Could you check a few things on this model? Use its own coordinates, in mm. Face numbers are marked on the shaded views. A direction names the side the tool comes from. Coordinates: 2 decimals unless noted, no trailing zeros. Loops run counter-clockwise (first coordinate to the right, second up) from the corner with the lowest first, then second, coordinate; pieces in that order, holes last. Notation, with made-up numbers: (46.25, 21) -> (66.25, 21) arc R15 ccw to (66.25, 47) -> close; hole circle Ø5 at (20, 33). An arc over 180 degrees is marked (long way). One line per question, with ' | ' between items. Start each with the question number.
(1) I'm going to push flat-ended pins straight in: pin 1 Ø8 at (x, z) = (-11, 19) entering from -Y; pin 2 Ø7 at (y, z) = (-12, -36) entering from +X; pin 3 Ø10 at (y, z) = (-12, 4.5) entering from +X; pin 4 Ø2 at (x, y) = (-43.5, -7.5) entering from -Z. Where does each tip first touch, or does it pass through?
(2) Suppose I cut it at C-C (y = -16.5). Please give me the cut outline in (x, z).
(3) If I drill on line 1 along Y through (x, z) = (-49.5, 34); line 2 along X through (y, z) = (-4.5, 5); line 3 along X through (y, z) = (-25.5, 32), over which ranges is the centre line in solid material (lowest first)?
(4) Suppose I cut it at D-D (z = -35.5). Please give me the cut outline in (x, y).
(5) If we mould it in two halves opening along Z, with no side actions, what happens to the marked faces 1, 2 and 3? For each: pulls with the +Z half, pulls with the -Z half, needs draft (parallel to the pull), parting line crosses it, or undercut.
(6) Which directions (+Z, -Z, +X, -X, +Y, -Y) give clear straight access to the entire face, cutting with the end or side of a thin tool? Please do the marked faces 4, 5, 6 and 7.
(7) Suppose I cut it at B-B (z = 31). Please give me the cut outline in (x, y).
(8) Suppose I cut it at A-A (y = -25). Please give me the cut outline in (x, z) (3 decimals).
```python
from build123d import *

# Parameters (mm, degrees)
F0_W         = 130.5194124579
F0_H         = 87.0954208076
F1_DEPTH     = 5.08
F2_W         = 18.4217169881
F2_H         = 20.1326627284
F3_DEPTH     = 25.4
F4_W         = 18.0227532983
F4_H         = 20.2161408961
F5_DEPTH     = 25.4
F6_W         = 17.5940208137
F6_H         = 28.6207161844
F7_DEPTH     = 25.4
F8_T         = 2.54
F8_T3_DEPTH  = 22.6740208137
F8_T5_DEPTH  = 23.1027532983
F8_T7_DEPTH  = 25.2961408961
F8_T9_DEPTH  = 23.5017169881
F8_T11_DEPTH = 25.2126627284
F9_W         = 15.0540208137
F9_H         = 4.0768496692
F10_DEPTH    = 5.08
F11_W        = 26.8854014575
F11_H        = 26.7390697263
F12_DEPTH    = 2.54
F13_T1_DEPTH = 48.8824467137
F13_T3_DEPTH = 48.7361149824


# Not quite as in the source:
# - a fillet or chamfer that OpenCascade refuses, or shapes differently, is made with other operations: its cross-section is extruded or revolved along the edge and cut away or added
# - a shell that OpenCascade refuses in one call is made with other operations: the cavity is built on its own and cut out


with BuildPart() as f1:
    # F0 (on Front) → F1 (new body)
    with BuildSketch(Plane.XZ):
        with Locations((2.1416731179, -2.8366688639)):
            Rectangle(F0_W, F0_H)
    extrude(amount=F1_DEPTH)

    # F2 (on face) → F3 (join)
    with BuildSketch(Plane.XZ.offset(5.08)):
        with Locations((-53.9071746171, 30.6447101757)):
            Rectangle(F2_W, F2_H)
    extrude(amount=F3_DEPTH)

    # F4 (on face) → F5 (join)
    with BuildSketch(Plane.XZ.offset(5.08)):
        with Locations((-54.106656462, 0.4099132493)):
            Rectangle(F4_W, F4_H)
    extrude(amount=F5_DEPTH)

    # F6 (on face) → F7 (join)
    with BuildSketch(Plane.XZ.offset(5.08)):
        with Locations((-54.3210227042, -32.0740211755)):
            Rectangle(F6_W, F6_H)
    extrude(amount=F7_DEPTH)

    # F8: shell of thickness 2.54, made by hand


with BuildPart() as f8_core1:
    # F8_t2: copy of F1
    add(f1.part)

    # the walls: a layer under each face that stays
    f8_faces = [f8_core1.faces().sort_by_distance(p)[0] for p in [
        (-63.1180331111, -15.24, -2.8366688639),
        (2.1416731179, 0, -2.8366688639),
        (67.4013793468, -2.54, -2.8366688639),
        (-53.7952179355, -28.3028571429, -46.3843792677),
        (-54.3210227042, -30.48, -32.0740211755),
        (-54.3210227042, -17.78, -17.7636630833),
        (-54.106656462, -17.78, -9.6981571987),
        (-45.0952798128, -17.78, 0.4099132493),
        (-54.106656462, -30.48, 0.4099132493),
        (-54.106656462, -17.78, 10.5179836974),
        (2.1416731179, -5.08, -2.8366688639),
        (-44.696316123, -17.78, 30.6447101757),
        (-53.9071746171, -17.78, 20.5783788115),
        (-53.9071746171, -30.48, 30.6447101757),
        (58.0785641713, -2.1771428571, 40.7110415399),
    ]]
    thicken(f8_faces, amount=-F8_T, mode=Mode.SUBTRACT)

    # F8_s4 → F8_t3 (cut)
    with BuildSketch(Plane.YZ.offset(-65.6580331111)):
        Polygon((-5.1054, -17.7382630833), (-5.08, -20.3036630833), (-2.54, -20.3036630833), (-2.54, -17.7636630833), align=None)
    extrude(amount=F8_T3_DEPTH, mode=Mode.SUBTRACT)

    # F8_s6 → F8_t5 (cut)
    with BuildSketch(Plane.YZ.offset(-65.6580331111)):
        Polygon((-5.1054, -9.7235571987), (-5.08, -7.1581571987), (-2.54, -7.1581571987), (-2.54, -9.6981571987), align=None)
        Polygon((-5.1054, 10.5433836974), (-5.08, 7.9779836974), (-2.54, 7.9779836974), (-2.54, 10.5179836974), align=None)
    extrude(amount=F8_T5_DEPTH, mode=Mode.SUBTRACT)

    # F8_s8 → F8_t7 (cut)
    with BuildSketch(Plane.XY.offset(-12.2381571987)):
        Polygon((-45.0698798128, -5.1054), (-47.6352798128, -5.08), (-47.6352798128, -2.54), (-45.0952798128, -2.54), align=None)
    extrude(amount=F8_T7_DEPTH, mode=Mode.SUBTRACT)

    # F8_s10 → F8_t9 (cut)
    with BuildSketch(Plane.YZ.offset(-65.6580331111)):
        Polygon((-5.1054, 20.5529788115), (-2.54, 20.5783788115), (-2.54, 23.1183788115), (-5.08, 23.1183788115), align=None)
    extrude(amount=F8_T9_DEPTH, mode=Mode.SUBTRACT)

    # F8_s12 → F8_t11 (cut)
    with BuildSketch(Plane.XY.offset(18.0383788115)):
        Polygon((-44.670916123, -5.1054), (-44.696316123, -2.54), (-47.236316123, -2.54), (-47.236316123, -5.08), align=None)
    extrude(amount=F8_T11_DEPTH, mode=Mode.SUBTRACT)


with BuildPart() as f1_1:
    add(f1.part)

    # what is left inside the walls is the cavity
    f8_cavity = [f8_core1.part.solids().sort_by_distance(p)[0] for p in [
        (-60.552633, -19.473333, 30.64471),
        (-60.552633, -19.473333, -32.074021),
        (-60.552633, -19.473333, 0.409913),
    ]]
    add(f8_cavity, mode=Mode.SUBTRACT)

    # F9 (on face) → F10 (join)
    with BuildSketch(Plane(origin=(0, -27.94, 0), x_dir=(-1, 0, 0), z_dir=(0, 1, 0))):
        with Locations((53.0510227042, -30.6365806609)):
            Rectangle(F9_W, F9_H)
    extrude(amount=F10_DEPTH)

    # F11 (on face) → F12 (join)
    with BuildSketch(Plane.XZ.offset(5.08)):
        with Locations((0, -3.7744471338)):
            Rectangle(F11_W, F11_H)
    extrude(amount=F12_DEPTH)

    # F13: fillet of radius 5.08 on 4 edges, made by hand

    # F13_s2 → F13_t1 (cut)
    with BuildSketch(Plane.YZ.offset(-24.4412233568)):
        with BuildLine():
            ThreePointArc((-5.08, -17.1439819969), (-6.9394090512, -15.2845729457), (-7.62, -12.7445729457))
            Line((-7.62, -12.7445729457), (-7.62, -17.1439819969))
            Line((-7.62, -17.1439819969), (-5.08, -17.1439819969))
        make_face()
        with BuildLine():
            ThreePointArc((-5.08, 9.5950877294), (-6.9394090512, 7.7356786782), (-7.62, 5.1956786782))
            Line((-7.62, 5.1956786782), (-7.62, 9.5950877294))
            Line((-7.62, 9.5950877294), (-5.08, 9.5950877294))
        make_face()
    extrude(amount=F13_T1_DEPTH, mode=Mode.SUBTRACT)

    # F13_s4 → F13_t3 (cut)
    with BuildSketch(Plane.XY.offset(-28.142504625)):
        with BuildLine():
            ThreePointArc((-13.4427007288, -5.08), (-11.5832916775, -6.9394090512), (-9.0432916775, -7.62))
            Line((-9.0432916775, -7.62), (-13.4427007288, -7.62))
            Line((-13.4427007288, -7.62), (-13.4427007288, -5.08))
        make_face()
        with BuildLine():
            ThreePointArc((13.4427007288, -5.08), (11.5832916775, -6.9394090512), (9.0432916775, -7.62))
            Line((9.0432916775, -7.62), (13.4427007288, -7.62))
            Line((13.4427007288, -7.62), (13.4427007288, -5.08))
        make_face()
    extrude(amount=F13_T3_DEPTH, mode=Mode.SUBTRACT)


solid = f1_1.part
```
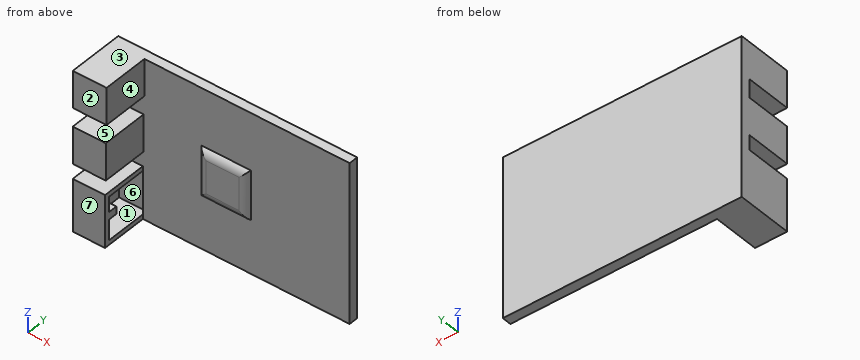
Checks:
1) pin 1: stops at y = -5.08 | pin 2: stops at x = -60.58 | pin 3: stops at x = 11.48 | pin 4: passes through
2) outline: (-63.12, -46.38) -> (-45.52, -46.38) -> (-45.52, -43.84) -> (-60.58, -43.84) -> (-60.58, -20.3) -> (-45.52, -20.3) -> (-45.52, -17.76) -> (-63.12, -17.76) -> close; (-63.12, -9.7) -> (-45.1, -9.7) -> (-45.1, 10.52) -> (-63.12, 10.52) -> close; (-63.12, 20.58) -> (-44.7, 20.58) -> (-44.7, 40.71) -> (-63.12, 40.71) -> close; hole (-60.58, -7.16) -> (-47.64, -7.16) -> (-47.64, 7.98) -> (-60.58, 7.98) -> close; hole (-60.58, 23.12) -> (-47.24, 23.12) -> (-47.24, 38.17) -> (-60.58, 38.17) -> close
3) line 1: y = -30.48 to -27.94, -2.54 to 0 | line 2: x = -63.12 to -60.58, -47.64 to 67.4 | line 3: x = -63.12 to -60.58, -47.24 to -44.7
4) outline: (-63.12, -30.48) -> (-45.52, -30.48) -> (-45.52, -27.94) -> (-60.58, -27.94) -> (-60.58, -2.54) -> (-45.52, -2.54) -> (-45.52, -5.08) -> (67.4, -5.08) -> (67.4, 0) -> (-63.12, 0) -> close
5) face 1: undercut | face 2: needs draft | face 3: pulls with the +Z half
6) face 4: +Z, -Z, +X, -Y | face 5: +X, -X, -Y | face 6: none | face 7: +Z, -Z, +X, -X, -Y
7) outline: (-63.12, -30.48) -> (-44.7, -30.48) -> (-44.7, -5.08) -> (67.4, -5.08) -> (67.4, 0) -> (-63.12, 0) -> close; hole (-60.58, -27.94) -> (-47.24, -27.94) -> (-47.24, -2.54) -> (-60.58, -2.54) -> close
8) outline: (-63.118, -46.384) -> (-45.524, -46.384) -> (-45.524, -43.844) -> (-60.578, -43.844) -> (-60.578, -32.675) -> (-45.524, -32.675) -> (-45.524, -28.598) -> (-60.578, -28.598) -> (-60.578, -20.304) -> (-45.524, -20.304) -> (-45.524, -17.764) -> (-63.118, -17.764) -> close; (-63.118, -9.698) -> (-45.095, -9.698) -> (-45.095, 10.518) -> (-63.118, 10.518) -> close; (-63.118, 20.578) -> (-44.696, 20.578) -> (-44.696, 40.711) -> (-63.118, 40.711) -> close; hole (-60.578, -7.158) -> (-47.635, -7.158) -> (-47.635, 7.978) -> (-60.578, 7.978) -> close; hole (-60.578, 23.118) -> (-47.236, 23.118) -> (-47.236, 38.171) -> (-60.578, 38.171) -> close
